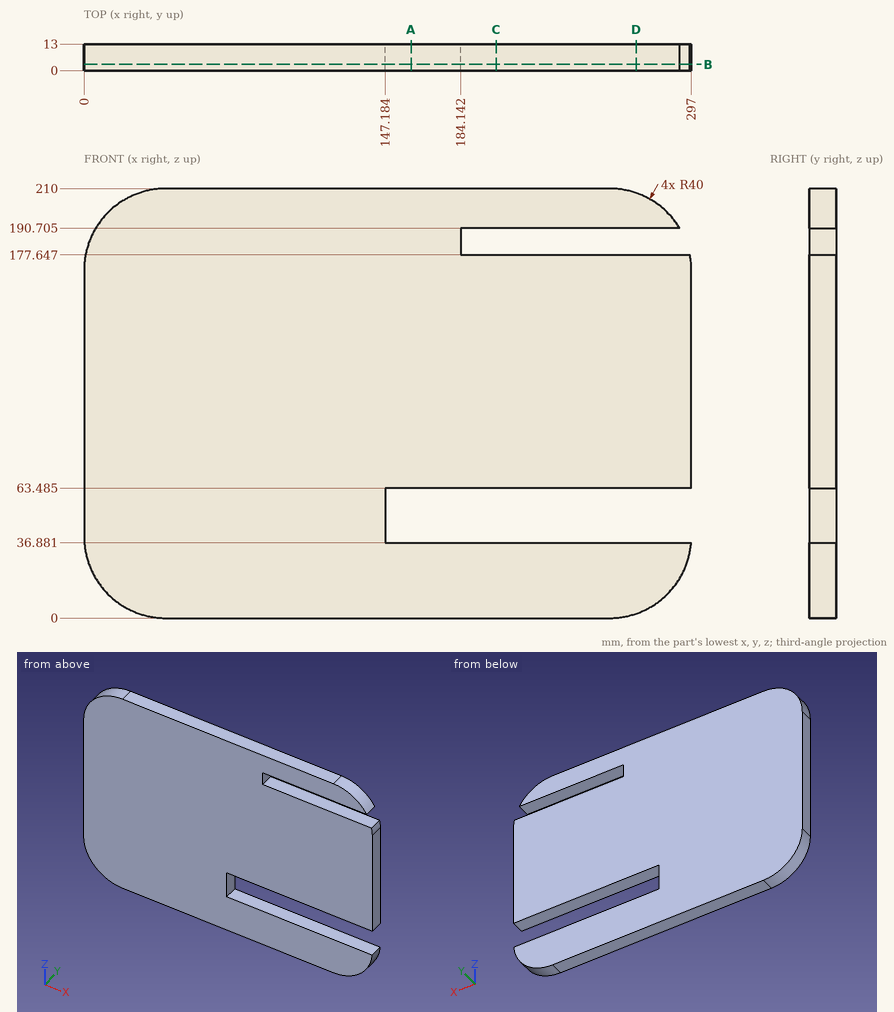
Input: dimensioned drawing with shaded views. Units: mm. Origin: part minimum x, y, z. Give positions to 0.01 mm unless a question says otherwise; leave off trailing zeros. Write each loop counter-clockwise with the first axis right and the second up, starting at its lowest first coordinate (ties: lowest second). Pieces come first, ordered by that corner, then holes. Notation, with made-up numbers: (-7, -19.75) - (10, -19.75) arc R18 cw to (10, 6.25) - close; hole circle Ø9 at (46.25, 5). An arc over 180 degrees is marked (long way). Write item = value, one per line. Start each with the question number.
1) Material intervals for L1, parallel to Z at x = 256.5, y = 0.5 (1 decimal); L2, parallel to Z at x = 269, y = 1.25 (1 decimal); L3, parallel to Z at x = 170, y = 10.75 (1 decimal), sorted ascending. Write a range as [from, to].
2) Cut plane B-B (y = 3). Return loops of the section in (x, z) (1 decimal), and give its area (3 significant figures).
3) Pin query (flat end, axial travel): pin 1 (6.5 mm diameter, centred on y = 5.5, z = 186.5, fed in from +X); pin 2 (1.5 mm diameter, centred on y = 1.5, z = 185.5, fed in from -X); pin 3 (2 mm diameter, centred on y = 1.5, z = 174.5, fed in from +X). Return the tip coordinate at first contact, or that it passes through.
4) Cut plane C-C (x = 201.5). Return loops of the section in (y, z) (1 decimal).
5) Cut plane D-D (x = 270). Return loops of the section in (y, z) (1 decimal).
6) Cut plane A-A (x = 160). Return loops of the section in (y, z) (1 decimal), and give its area (3 significant figures).
Answers follow:
q1.L1 = [0, 36.9], [63.5, 177.6], [190.7, 210]
q1.L2 = [1.8, 36.9], [63.5, 177.6], [190.7, 208.2]
q1.L3 = [0, 36.9], [63.5, 210]
q2.outline = (0, 40) arc R40 ccw to (40, 0) - (257, 0) arc R40 ccw to (296.9, 36.9) - (147.2, 36.9) - (147.2, 63.5) - (297, 63.5) - (297, 170) arc R40 ccw to (296.3, 177.6) - (184.1, 177.6) - (184.1, 190.7) - (291.2, 190.7) arc R40 ccw to (257, 210) - (40, 210) arc R40 ccw to (0, 170) - close
q2.area = 55,600 mm^2
q3.pin_1 = 184.14
q3.pin_2 = 2.82
q3.pin_3 = 296.85
q4.outline = (0, 0) - (13, 0) - (13, 36.9) - (0, 36.9) - close; (0, 63.5) - (13, 63.5) - (13, 177.6) - (0, 177.6) - close; (0, 190.7) - (13, 190.7) - (13, 210) - (0, 210) - close
q5.outline = (0, 2.2) - (13, 2.2) - (13, 36.9) - (0, 36.9) - close; (0, 63.5) - (13, 63.5) - (13, 177.6) - (0, 177.6) - close; (0, 190.7) - (13, 190.7) - (13, 207.8) - (0, 207.8) - close
q6.outline = (0, 0) - (13, 0) - (13, 36.9) - (0, 36.9) - close; (0, 63.5) - (13, 63.5) - (13, 210) - (0, 210) - close
q6.area = 2,380 mm^2
